Read the model definition and answer for the solid it produces. Units are mm, in the model's axes. A direction names the side the tool comes from. Give positions to 0.01 mm unless a question says otherwise; leave off trailing zeros. Write each loop counter-clockwise with the first axis right and the second up, starting at its lowest first coordinate (ties: lowest second). Pieces come first, ordered by that corner, then holes. Notation, with made-up numbers: M 24,24.25 L 41,24.25 A26 cw 41,56.25 Z; hole C 81.5,85 d7. An arc over 180 degrees is marked long. Use a Markdown table: item, result. Add a question column.
Item 1: A cutting plane is placed at D-D on x = -16. Determine the outline of the cut face in (y, z), then the cut area to 3 significant figures.
Item 2: For faces 1 (the flat face through (-16, -8.577, 1)), 2 (the flat face through (0, 24.5, 1)), determine the directions among +Z, -Z, +X, -X, +Y, -Y from which every point of the face is accessible in a straight line to the end or side of a thin tool.
Item 3: A cutting plane is placed at A-A on y = 1. Determine the outline of the cut face in (x, z), then the cut area to 3 significant figures.
Item 4: Consider probe 1 along Y at (x, z) = (17.5, 1.15); probe 2 along X at (y, z) = (15.5, 0.5); probe 3 along Y at (x, z) = (-5, 1.25). Determine where each line is inside the solid, lowest interval first. Write a range as [from, to].
Item 5: A cutting plane is placed at B-B on y = -17.5. Determine the outline of the cut face in (x, z).
from build123d import *

# Parameters (mm, degrees)
SKETCH1_W           = 49
SKETCH1_H           = 49
SKETCH1_R           = 2.2
BOSS_EXTRUDE1_DEPTH = 3
SKETCH2_R           = 1.55
SKETCH2_R_2         = 1.5
SKETCH2_W           = 3.699471197
SKETCH2_H           = 15.29419199
CUT_EXTRUDE1_DEPTH  = 3


with BuildPart() as part:
    # Sketch1 → Boss-Extrude1 (new body)
    with BuildSketch(Plane.XY):
        Rectangle(SKETCH1_W, SKETCH1_H)
        with Locations((-17.5, -17.5)):
            Circle(SKETCH1_R, mode=Mode.SUBTRACT)
        with Locations((17.5, 17.5)):
            Circle(SKETCH1_R, mode=Mode.SUBTRACT)
        with Locations((17.5, -17.5)):
            Circle(SKETCH1_R, mode=Mode.SUBTRACT)
        with Locations((-17.5, 17.5)):
            Circle(SKETCH1_R, mode=Mode.SUBTRACT)
    extrude(amount=BOSS_EXTRUDE1_DEPTH)

    # Sketch2 → Cut-Extrude1 (cut)
    with BuildSketch(Plane(origin=(0, 0, 0), x_dir=(-1, 0, 0), z_dir=(0, 0, -1))):
        with Locations((-6.717514421, 6.717514421)):
            Circle(SKETCH2_R)
        with Locations((5.656854249, 5.656854249)):
            Circle(SKETCH2_R_2)
        with Locations((6.717514421, -6.717514421)):
            Circle(SKETCH2_R)
        with Locations((-5.656854249, -5.656854249)):
            Circle(SKETCH2_R_2)
        with Locations((15.650264401, -0.929581574)):
            Rectangle(SKETCH2_W, SKETCH2_H)
    extrude(amount=-CUT_EXTRUDE1_DEPTH, mode=Mode.SUBTRACT)


solid = part.part
Filled in:
| question | item | result |
|---|---|---|
| 1 | outline | M -24.5,0 L -19.11,0 L -19.11,3 L -24.5,3 Z; M -15.89,0 L -8.58,0 L -8.58,3 L -15.89,3 Z; M 6.72,0 L 15.89,0 L 15.89,3 L 6.72,3 Z; M 19.11,0 L 24.5,0 L 24.5,3 L 19.11,3 Z |
| 1 | area | 81.8 mm² |
| 2 | face 1 | +Z, -Z |
| 2 | face 2 | +Z, -Z, +X, -X, +Y |
| 3 | outline | M -24.5,0 L -17.5,0 L -17.5,3 L -24.5,3 Z; M -13.8,0 L 24.5,0 L 24.5,3 L -13.8,3 Z |
| 3 | area | 136 mm² |
| 4 | probe 1 | [-24.5, -19.7], [-15.3, 15.3], [19.7, 24.5] |
| 4 | probe 2 | [-24.5, -18.42], [-16.58, 16.58], [18.42, 24.5] |
| 4 | probe 3 | [-24.5, 4.31], [7.01, 24.5] |
| 5 | outline | M -24.5,0 L -19.7,0 L -19.7,3 L -24.5,3 Z; M -15.3,0 L 15.3,0 L 15.3,3 L -15.3,3 Z; M 19.7,0 L 24.5,0 L 24.5,3 L 19.7,3 Z |
